Verification items for the finished model (mm, model axes). A direction names the side the tool comes from. Round coordinates to 2 decimals unless told otherwise and drop trailing zeros. Order: outer loops, then holes, each group sorted by start corner. A loop starts at its lowest first (then second) coordinate and runs counter-clockwise, first axis right, second up. Notation, with made-up numbers: (77.25, -22) -> (126.25, -22) arc R14 cw to (126.25, 1) -> close; hole circle Ø6 at (-4, -19.5). An arc over 180 degrees is marked (long way). Put each result on its own line as item: value.
from build123d import *

# Parameters (mm, degrees)
F0_R     = 90
F0_W     = 30
F0_H     = 0.5
F0_R_2   = 3.17
F1_DEPTH = 3


with BuildPart() as f1:
    # F0 (on Front) → F1 (new body)
    with BuildSketch(Plane.XZ):
        Circle(F0_R)
        with BuildLine():
            ThreePointArc((-41.078762, -77.257914), (-45.686982, -74.625396), (-50.127129, -71.718345))
            ThreePointArc((-50.127129, -71.718345), (-50.979425, -70.167154), (-50.266941, -68.546979))
            Line((-50.266941, -68.546979), (-44.332839, -63.567676))
            ThreePointArc((-44.332839, -63.567676), (-44.12, -63.715584), (-43.906667, -63.862779))
            Line((-43.906667, -63.862779), (-49.945547, -68.930001))
            ThreePointArc((-49.945547, -68.930001), (-50.47991, -70.145133), (-49.840688, -71.308525))
            ThreePointArc((-49.840688, -71.308525), (-45.425914, -74.198965), (-40.844026, -76.816441))
            Line((-40.844026, -76.816441), (-41.078762, -77.257914))
        make_face(mode=Mode.SUBTRACT)
        with BuildLine():
            Line((-29.926763, -82.223104), (-29.755752, -81.753258))
            ThreePointArc((-29.755752, -81.753258), (-18.088317, -85.098841), (-6.068813, -86.788072))
            Line((-6.068813, -86.788072), (-6.103691, -87.286854))
            ThreePointArc((-6.103691, -87.286854), (-18.192273, -85.587915), (-29.926763, -82.223104))
        make_face(mode=Mode.SUBTRACT)
        Polygon((-20.795181, -76.835932), (-20.408811, -76.93946), (-21.702906, -81.769089), (-22.089276, -81.665561), align=None, mode=Mode.SUBTRACT)
        with BuildLine():
            Line((6.103691, -87.286854), (6.068813, -86.788072))
            ThreePointArc((6.068813, -86.788072), (18.088317, -85.098841), (29.755752, -81.753258))
            Line((29.755752, -81.753258), (29.926763, -82.223104))
            ThreePointArc((29.926763, -82.223104), (18.192273, -85.587915), (6.103691, -87.286854))
        make_face(mode=Mode.SUBTRACT)
        Polygon((22.089276, -81.665561), (21.702906, -81.769089), (20.408811, -76.93946), (20.795181, -76.835932), align=None, mode=Mode.SUBTRACT)
        with BuildLine():
            ThreePointArc((50.266941, -68.546979), (50.979425, -70.167154), (50.127129, -71.718345))
            ThreePointArc((50.127129, -71.718345), (45.686982, -74.625396), (41.078762, -77.257914))
            Line((41.078762, -77.257914), (40.844026, -76.816441))
            ThreePointArc((40.844026, -76.816441), (45.425914, -74.198965), (49.840688, -71.308525))
            ThreePointArc((49.840688, -71.308525), (50.47991, -70.145133), (49.945547, -68.930001))
            Line((49.945547, -68.930001), (43.906667, -63.862779))
            ThreePointArc((43.906667, -63.862779), (44.12, -63.715584), (44.332839, -63.567676))
            Line((44.332839, -63.567676), (50.266941, -68.546979))
        make_face(mode=Mode.SUBTRACT)
        with BuildLine():
            Line((-23.722514, -46.27356), (-20.714425, -43.749474))
            ThreePointArc((-20.714425, -43.749474), (-20.187384, -43.062621), (-20, -42.217385))
            Line((-20, -42.217385), (-20, -35.15))
            Line((-20, -35.15), (-19.5, -35.15))
            Line((-19.5, -35.15), (-19.5, -25.15))
            Line((-19.5, -25.15), (-20, -25.15))
            Line((-20, -25.15), (-20, -15.15))
            Line((-20, -15.15), (-20, -13.15))
            Line((-20, -13.15), (-18, -13.15))
            Line((-18, -13.15), (-7.5, -13.15))
            Line((-7.5, -13.15), (7.5, -13.15))
            Line((7.5, -13.15), (18, -13.15))
            Line((18, -13.15), (20, -13.15))
            Line((20, -13.15), (20, -15.15))
            Line((20, -15.15), (20, -25.15))
            Line((20, -25.15), (19.5, -25.15))
            Line((19.5, -25.15), (19.5, -35.15))
            Line((19.5, -35.15), (20, -35.15))
            Line((20, -35.15), (20, -42.217385))
            ThreePointArc((20, -42.217385), (20.187384, -43.062621), (20.714425, -43.749474))
            Line((20.714425, -43.749474), (23.722514, -46.27356))
            ThreePointArc((23.722514, -46.27356), (23.480225, -46.396972), (23.237294, -46.519116))
            Line((23.237294, -46.519116), (20.393031, -44.132496))
            ThreePointArc((20.393031, -44.132496), (19.976222, -43.685146), (19.680468, -43.15))
            Line((19.680468, -43.15), (-19.680468, -43.15))
            ThreePointArc((-19.680468, -43.15), (-19.976222, -43.685146), (-20.393031, -44.132496))
            Line((-20.393031, -44.132496), (-23.237294, -46.519116))
            ThreePointArc((-23.237294, -46.519116), (-23.480225, -46.396972), (-23.722514, -46.27356))
        make_face(mode=Mode.SUBTRACT)
        with Locations((0, -9.15)):
            Rectangle(F0_W, F0_H, mode=Mode.SUBTRACT)
        with BuildLine():
            Line((-49.945547, 68.930001), (-43.906667, 63.862779))
            ThreePointArc((-43.906667, 63.862779), (-44.12, 63.715584), (-44.332839, 63.567676))
            Line((-44.332839, 63.567676), (-50.266941, 68.546979))
            ThreePointArc((-50.266941, 68.546979), (-50.979425, 70.167154), (-50.127129, 71.718345))
            ThreePointArc((-50.127129, 71.718345), (-45.686982, 74.625396), (-41.078762, 77.257914))
            Line((-41.078762, 77.257914), (-40.844026, 76.816441))
            ThreePointArc((-40.844026, 76.816441), (-45.425914, 74.198965), (-49.840688, 71.308525))
            ThreePointArc((-49.840688, 71.308525), (-50.47991, 70.145133), (-49.945547, 68.930001))
        make_face(mode=Mode.SUBTRACT)
        Polygon((-22.089276, 81.665561), (-21.702906, 81.769089), (-20.408811, 76.93946), (-20.795181, 76.835932), align=None, mode=Mode.SUBTRACT)
        with BuildLine():
            ThreePointArc((-6.068813, 86.788072), (-18.088317, 85.098841), (-29.755752, 81.753258))
            Line((-29.755752, 81.753258), (-29.926763, 82.223104))
            ThreePointArc((-29.926763, 82.223104), (-18.192273, 85.587915), (-6.103691, 87.286854))
            Line((-6.103691, 87.286854), (-6.068813, 86.788072))
        make_face(mode=Mode.SUBTRACT)
        Circle(F0_R_2, mode=Mode.SUBTRACT)
        with Locations((0, 9.15)):
            Rectangle(F0_W, F0_H, mode=Mode.SUBTRACT)
        with BuildLine():
            ThreePointArc((19.680468, 43.15), (19.976222, 43.685146), (20.393031, 44.132496))
            Line((20.393031, 44.132496), (23.237294, 46.519116))
            ThreePointArc((23.237294, 46.519116), (23.480225, 46.396972), (23.722514, 46.27356))
            Line((23.722514, 46.27356), (20.714425, 43.749474))
            ThreePointArc((20.714425, 43.749474), (20.187384, 43.062621), (20, 42.217385))
            Line((20, 42.217385), (20, 35.15))
            Line((20, 35.15), (19.5, 35.15))
            Line((19.5, 35.15), (19.5, 25.15))
            Line((19.5, 25.15), (20, 25.15))
            Line((20, 25.15), (20, 15.15))
            Line((20, 15.15), (20, 13.15))
            Line((20, 13.15), (18, 13.15))
            Line((18, 13.15), (7.5, 13.15))
            Line((7.5, 13.15), (-7.5, 13.15))
            Line((-7.5, 13.15), (-18, 13.15))
            Line((-18, 13.15), (-20, 13.15))
            Line((-20, 13.15), (-20, 15.15))
            Line((-20, 15.15), (-20, 25.15))
            Line((-20, 25.15), (-19.5, 25.15))
            Line((-19.5, 25.15), (-19.5, 35.15))
            Line((-19.5, 35.15), (-20, 35.15))
            Line((-20, 35.15), (-20, 42.217385))
            ThreePointArc((-20, 42.217385), (-20.187384, 43.062621), (-20.714425, 43.749474))
            Line((-20.714425, 43.749474), (-23.722514, 46.27356))
            ThreePointArc((-23.722514, 46.27356), (-23.480225, 46.396972), (-23.237294, 46.519116))
            Line((-23.237294, 46.519116), (-20.393031, 44.132496))
            ThreePointArc((-20.393031, 44.132496), (-19.976222, 43.685146), (-19.680468, 43.15))
            Line((-19.680468, 43.15), (19.680468, 43.15))
        make_face(mode=Mode.SUBTRACT)
        Polygon((20.795181, 76.835932), (20.408811, 76.93946), (21.702906, 81.769089), (22.089276, 81.665561), align=None, mode=Mode.SUBTRACT)
        with BuildLine():
            Line((29.926763, 82.223104), (29.755752, 81.753258))
            ThreePointArc((29.755752, 81.753258), (18.088317, 85.098841), (6.068813, 86.788072))
            Line((6.068813, 86.788072), (6.103691, 87.286854))
            ThreePointArc((6.103691, 87.286854), (18.192273, 85.587915), (29.926763, 82.223104))
        make_face(mode=Mode.SUBTRACT)
        with BuildLine():
            ThreePointArc((44.332839, 63.567676), (44.12, 63.715584), (43.906667, 63.862779))
            Line((43.906667, 63.862779), (49.945547, 68.930001))
            ThreePointArc((49.945547, 68.930001), (50.47991, 70.145133), (49.840688, 71.308525))
            ThreePointArc((49.840688, 71.308525), (45.425914, 74.198965), (40.844026, 76.816441))
            Line((40.844026, 76.816441), (41.078762, 77.257914))
            ThreePointArc((41.078762, 77.257914), (45.686982, 74.625396), (50.127129, 71.718345))
            ThreePointArc((50.127129, 71.718345), (50.979425, 70.167154), (50.266941, 68.546979))
            Line((50.266941, 68.546979), (44.332839, 63.567676))
        make_face(mode=Mode.SUBTRACT)
    extrude(amount=F1_DEPTH)


solid = f1.part
Item 1: Section check C-C on y = -2.4. State how many separate pieces and enclosed holes the cut face has, then the cut area to 3 significant figures.
Check sheet entries:
separate pieces: 1
enclosed holes: 17
area: 22,900 mm^2
Item 2: Material ranges on L1, parallel to Z at x = 0, y = -0.7; L2, parallel to Z at x = 24.5, y = -2.5; L3, parallel to Z at x = -25, y = -1.65, recorded low to high. Write a range as [from, to].
Check sheet entries:
L1: z = [-90, -43.15], [-13.15, -9.4], [-8.9, -3.17], [3.17, 8.9], [9.4, 13.15], [43.15, 90]
L2: z = [-86.6, -84], [-83.48, 83.48], [84, 86.6]
L3: z = [-86.46, -83.85], [-83.33, 83.33], [83.85, 86.46]
Item 3: Release check for a two-part mould opening along X. For faces 1 (the cylindrical face through (45.49, -1.48, 74.16)), 2 (the flat face through (19, 0, 1)), 3 (the cylindrical face through (-18.255, -1.479, -85.063)) record: +X half, -X half, draft (parallel to the pull), parting line (faces both ways), or undercut.
Check sheet entries:
face 1: undercut
face 2: draft
face 3: undercut
Item 4: Section check A-A on z = 0. Record the boundary of the cut face in (x, y).
Check sheet entries:
outline: (-90, -3) -> (-3.17, -3) -> (-3.17, 0) -> (-90, 0) -> close; (3.17, -3) -> (90, -3) -> (90, 0) -> (3.17, 0) -> close
Item 5: Section check D-D on x = 34. Record the boundary of the cut face in (y, z).
Check sheet entries:
outline: (-3, -83.33) -> (0, -83.33) -> (0, 83.33) -> (-3, 83.33) -> close
Item 6: Gauge pin test, flat ends, axial feed: pin 1 Ø0.9 at (x, y) = (4.5, -2) entering from +Z; pin 2 Ø0.9 at (y, z) = (-1.5, 38.5) entering from -X; pin 3 Ø1.5 at (x, y) = (-32.5, -1.5) entering from -Z. Record the tip position at first contact, or that the pin passes through.
Check sheet entries:
pin 1: stops at z = 89.91
pin 2: stops at x = -81.56
pin 3: stops at z = -84.21
Item 7: Tool access check on faces 4 (the flat face through (19, -3, 1)), 5 (the cylindrical face through (45.36, -1.48, -74.24)). Record the directions out of +Z, -Z, +X, -X, +Y, -Y that give a thin tool (end or side, any length) a straight path to the whole face; none if there is none.
Check sheet entries:
face 4: +Z, -Z, +X, -X, -Y
face 5: +Y, -Y
Item 8: Section check B-B on x = 0. Record the boundary of the cut face in (y, z), then the cut area to 3 significant figures.
Check sheet entries:
outline: (-3, -90) -> (0, -90) -> (0, -43.15) -> (-3, -43.15) -> close; (-3, -13.15) -> (0, -13.15) -> (0, -9.4) -> (-3, -9.4) -> close; (-3, -8.9) -> (0, -8.9) -> (0, -3.17) -> (-3, -3.17) -> close; (-3, 3.17) -> (0, 3.17) -> (0, 8.9) -> (-3, 8.9) -> close; (-3, 9.4) -> (0, 9.4) -> (0, 13.15) -> (-3, 13.15) -> close; (-3, 43.15) -> (0, 43.15) -> (0, 90) -> (-3, 90) -> close
area: 338 mm^2
